Model file for the job. Use its own axes, mm. A direction names the side the tool comes from. Coordinates: 2 decimals unless noted, no trailing zeros. Order: outer loops, then holes, each group sorted by start corner. A loop starts at its lowest first (then second) coordinate and runs counter-clockwise, first axis right, second up. Notation, with made-up numbers: (-20, 14.25) -> (12, 14.25) arc R30 cw to (12, 39.25) -> close; hole circle Ø3 at (12.5, 89). An arc over 180 degrees is marked (long way). Write item = value, one per line. Start each with the question number.
Q1. Cut at D-D, the plane y = 5. Give the number of separate pieces and of enclosed holes in the cut face, plus the area to 3 significant figures.
Q2. Cut at C-C, the plane z = 6. List the corners of the cut face in (x, y), plus the area to 3 significant figures.
Q3. 3-axis set-ups, long thin cutter, end or side, ignore diameter. For faces 5 (the face through (-16.5, 17, 12)), 6 (the face through (-13, 15.1, 19)), 7 (the face through (-13, 57.6, 9)): which of +Z, -Z, +X, -X, +Y, -Y reach the whole face in a straight line?
Q4. Mould opens along X. For faces 1 (the face through (-36.35, 3.97, 0.86)), 2 (the face through (16.7, 63, 9)), 3 (the face through (13, 22.7, 12)), 4 (the face through (13, 17, 15.85)) say: +X half, -X half, draft (parallel to the pull), parting line (faces both ways), or undercut.
Q5. Wall check: line 1 (Y direction, x = 35, z = 0.55); line 2 (X direction, y = 19, z = 19.5); line 3 (X direction, y = 105, z = 0.55). Give the ranges that are in metal, low to high. Write a range as from..to.
Q6. Cut at B-B, the plane y = 27.7. List the corners of the cut face in (x, z), plus the area to 3 significant figures.
Q7. Cut at A-A, the plane z = 11. List the corners of the cut face in (x, y), plus the area to 3 significant figures.
Q8. Flat gauge pins, fed straight in: pin 1 (4 mm diameter, centred on x = -14.5, y = 47, fed in from +Z); pin 2 (4.5 mm diameter, centred on x = 13.5, y = 63, fed in from +Z); pin 3 (1.6 mm diameter, centred on y = 18, z = 18, fed in from -X); pin 4 (2.5 mm diameter, centred on x = -11.667, y = 105, fed in from +Z). Where does each tip first touch, or does it go through?
from build123d import *

# Parameters (mm, degrees)
SKETCH014_W     = 80
SKETCH014_H     = 110
PAD004_DEPTH    = 3
SKETCH015_R     = 3.2
PAD005_DEPTH    = 1
SKETCH016_R     = 1.65
POCKET010_DEPTH = 4.001
SKETCH017_W     = 7.6
SKETCH017_H     = 10.6
PAD006_DEPTH    = 12.8
SKETCH018_W     = 5.2
SKETCH018_H     = 8.2
POCKET011_DEPTH = 8.2
SKETCH019_R     = 1.1
SKETCH019_R_2   = 1.7
POCKET012_DEPTH = 3.001
SKETCH020_W     = 6
SKETCH020_H     = 11
PAD007_DEPTH    = 18.55
SKETCH021_R     = 1.35
POCKET013_DEPTH = 56.501
SKETCH022_W     = 2.2
SKETCH022_H     = 5.2
POCKET014_DEPTH = 5.7
SKETCH023_R     = 1.1
POCKET015_DEPTH = 15.851
CHAMFER_SIZE    = 1
CHAMFER001_SIZE = 1.3
CHAMFER002_SIZE = 1
CHAMFER003_SIZE = 0.75
CHAMFER004_SIZE = 0.5


with BuildPart() as part:
    # Sketch014 → Pad004 (new body)
    with BuildSketch(Plane.XY):
        with Locations((0, 55)):
            Rectangle(SKETCH014_W, SKETCH014_H)
    extrude(amount=PAD004_DEPTH)

    # Sketch015 (on Face6 of Pad004) → Pad005 (join)
    with BuildSketch(Plane.XY.offset(3)):
        with Locations((0, 27.7)):
            Circle(SKETCH015_R)
    extrude(amount=PAD005_DEPTH)

    # Sketch016 (on Face8 of Pad005) → Pocket010 (cut, through all)
    with BuildSketch(Plane.XY.offset(4)):
        with Locations((0, 27.7)):
            Circle(SKETCH016_R)
    extrude(amount=-POCKET010_DEPTH, mode=Mode.SUBTRACT)

    # Sketch017 (on Face5 of Pocket010) → Pad006 (join)
    with BuildSketch(Plane.XY.offset(3)):
        with Locations((-12.9, 62.9)):
            Rectangle(SKETCH017_W, SKETCH017_H)
        with Locations((12.9, 62.9)):
            Rectangle(SKETCH017_W, SKETCH017_H)
    extrude(amount=PAD006_DEPTH)

    # Sketch018 (on Face18 of Pad006) → Pocket011 (cut)
    with BuildSketch(Plane.XY.offset(15.8)):
        with Locations((-12.9, 62.9)):
            Rectangle(SKETCH018_W, SKETCH018_H)
        with Locations((12.9, 62.9)):
            Rectangle(SKETCH018_W, SKETCH018_H)
    extrude(amount=-POCKET011_DEPTH, mode=Mode.SUBTRACT)

    # Sketch019 (on Face5 of Pocket011) → Pocket012 (cut, through all)
    with BuildSketch(Plane.XY.offset(3)):
        with Locations((0, 54)):
            Circle(SKETCH019_R)
        with Locations((-11.667, 5)):
            Circle(SKETCH019_R_2)
        with Locations((11.666, 5)):
            Circle(SKETCH019_R_2)
        with Locations((35, 5)):
            Circle(SKETCH019_R_2)
        with Locations((-35, 38.333)):
            Circle(SKETCH019_R_2)
        with Locations((-35, 71.666)):
            Circle(SKETCH019_R_2)
        with Locations((-35, 105)):
            Circle(SKETCH019_R_2)
        with Locations((35, 38.333)):
            Circle(SKETCH019_R_2)
        with Locations((35, 71.666)):
            Circle(SKETCH019_R_2)
        with Locations((35, 105)):
            Circle(SKETCH019_R_2)
        with Locations((-11.667, 105)):
            Circle(SKETCH019_R_2)
        with Locations((11.666, 105)):
            Circle(SKETCH019_R_2)
        with Locations((-35, 5)):
            Circle(SKETCH019_R_2)
    extrude(amount=-POCKET012_DEPTH, mode=Mode.SUBTRACT)

    # Sketch020 (on Face5 of Pocket012) → Pad007 (join)
    with BuildSketch(Plane.XY.offset(3)):
        with Locations((13.5, 17.2)):
            Rectangle(SKETCH020_W, SKETCH020_H)
        with Locations((-13.5, 17.2)):
            Rectangle(SKETCH020_W, SKETCH020_H)
    extrude(amount=PAD007_DEPTH)

    # Sketch021 (on Face22 of Pad007) → Pocket013 (cut, through all)
    with BuildSketch(Plane(origin=(-16.5, 0, 0), x_dir=(0, -1, 0), z_dir=(-1, 0, 0))):
        with Locations((-17.7, 18.675)):
            Circle(SKETCH021_R)
        Polygon((-11.7, 3.05), (-11.7, 21.6), (-13.1, 21.6), align=None)
    extrude(amount=-POCKET013_DEPTH, mode=Mode.SUBTRACT)

    # Sketch022 (on Face39 of Pocket013) → Pocket014 (cut)
    with BuildSketch(Plane.XY.offset(21.55)):
        with Locations((-13.4, 17.7)):
            Rectangle(SKETCH022_W, SKETCH022_H)
        with Locations((13.4, 17.7)):
            Rectangle(SKETCH022_W, SKETCH022_H)
    extrude(amount=-POCKET014_DEPTH, mode=Mode.SUBTRACT)

    # Sketch023 (on Face65 of Pocket014) → Pocket015 (cut, through all)
    with BuildSketch(Plane.XY.offset(15.85)):
        with Locations((13.4, 19)):
            Circle(SKETCH023_R)
        with Locations((-13.4, 19)):
            Circle(SKETCH023_R)
    extrude(amount=-POCKET015_DEPTH, mode=Mode.SUBTRACT)

    # Chamfer
    chamfer_edges = [part.edges().sort_by_distance(p)[0] for p in [
        (0, 0, 3),
        (40, 55, 3),
        (0, 110, 3),
        (-40, 55, 3),
        (-40, 0, 1.5),
        (40, 0, 1.5),
        (-40, 110, 1.5),
        (40, 110, 1.5),
    ]]
    chamfer(chamfer_edges, length=CHAMFER_SIZE)

    # Chamfer001
    chamfer001_edges = [part.edges().sort_by_distance(p)[0] for p in [
        (33.3, 5, 3),
        (33.3, 38.333, 3),
        (33.3, 71.666, 3),
        (33.3, 105, 3),
        (9.966, 105, 3),
        (-13.367, 105, 3),
        (-36.7, 105, 3),
        (-36.7, 71.666, 3),
        (-36.7, 38.333, 3),
        (-36.7, 5, 3),
        (-13.367, 5, 3),
        (9.966, 5, 3),
    ]]
    chamfer(chamfer001_edges, length=CHAMFER001_SIZE)

    # Chamfer002
    chamfer002_edges = [part.edges().sort_by_distance(p)[0] for p in [
        (-16.5, 17.898113, 21.55),
        (-13.5, 13.096226, 21.55),
        (-10.5, 17.898113, 21.55),
        (-13.5, 22.7, 21.55),
        (10.5, 17.898113, 21.55),
        (13.5, 13.096226, 21.55),
        (16.5, 17.898113, 21.55),
        (13.5, 22.7, 21.55),
        (16.7, 62.9, 15.8),
        (12.9, 68.2, 15.8),
        (9.1, 62.9, 15.8),
        (12.9, 57.6, 15.8),
        (-9.1, 62.9, 15.8),
        (-12.9, 68.2, 15.8),
        (-16.7, 62.9, 15.8),
        (-12.9, 57.6, 15.8),
    ]]
    chamfer(chamfer002_edges, length=CHAMFER002_SIZE)

    # Chamfer003
    chamfer003_edges = [part.edges().sort_by_distance(p)[0] for p in [
        (-1.1, 54, 3),
    ]]
    chamfer(chamfer003_edges, length=CHAMFER003_SIZE)

    # Chamfer004
    chamfer004_edges = [part.edges().sort_by_distance(p)[0] for p in [
        (-3.2, 27.7, 4),
    ]]
    chamfer(chamfer004_edges, length=CHAMFER004_SIZE)


solid = part.part
Here are the results:
q1.separate_pieces = 5
q1.enclosed_holes = 0
q1.area = 191 mm²
q2.outline = (-16.7, 57.6) -> (-9.1, 57.6) -> (-9.1, 68.2) -> (-16.7, 68.2) -> close; (-16.5, 11.92) -> (-10.5, 11.92) -> (-10.5, 22.7) -> (-16.5, 22.7) -> close; (9.1, 57.6) -> (16.7, 57.6) -> (16.7, 68.2) -> (9.1, 68.2) -> close; (10.5, 11.92) -> (16.5, 11.92) -> (16.5, 22.7) -> (10.5, 22.7) -> close; hole circle Ø2.2 at (-13.4, 19); hole circle Ø2.2 at (13.4, 19)
q2.area = 283 mm²
q3.face_5 = +Z, -X, -Y
q3.face_6 = +Z
q3.face_7 = +Z, +X, -X
q4.face_1 = undercut
q4.face_2 = +X half
q4.face_3 = draft
q4.face_4 = undercut
q5.line_1 = 0..3.3, 6.7..36.63, 40.03..69.97, 73.37..103.3, 106.7..110
q5.line_2 = -16.5..-14.5, -12.3..-10.5, 10.5..12.3, 14.5..16.5
q5.line_3 = -40..-36.7, -33.3..-13.37, -9.97..9.97, 13.37..33.3, 36.7..40
q6.outline = (-40, 0) -> (-1.65, 0) -> (-1.65, 4) -> (-2.7, 4) -> (-3.2, 3.5) -> (-3.2, 3) -> (-39, 3) -> (-40, 2) -> close; (1.65, 0) -> (40, 0) -> (40, 2) -> (39, 3) -> (3.2, 3) -> (3.2, 3.5) -> (2.7, 4) -> (1.65, 4) -> close
q6.area = 232 mm²
q7.outline = (-16.7, 57.6) -> (-9.1, 57.6) -> (-9.1, 68.2) -> (-16.7, 68.2) -> close; (-16.5, 12.3) -> (-10.5, 12.3) -> (-10.5, 22.7) -> (-16.5, 22.7) -> close; (9.1, 57.6) -> (16.7, 57.6) -> (16.7, 68.2) -> (9.1, 68.2) -> close; (10.5, 12.3) -> (16.5, 12.3) -> (16.5, 22.7) -> (10.5, 22.7) -> close; hole (-15.5, 58.8) -> (-10.3, 58.8) -> (-10.3, 67) -> (-15.5, 67) -> close; hole circle Ø2.2 at (-13.4, 19); hole (10.3, 58.8) -> (15.5, 58.8) -> (15.5, 67) -> (10.3, 67) -> close; hole circle Ø2.2 at (13.4, 19)
q7.area = 193 mm²
q8.pin_1 = 3
q8.pin_2 = 15.8
q8.pin_3 = -16.5
q8.pin_4 = through
